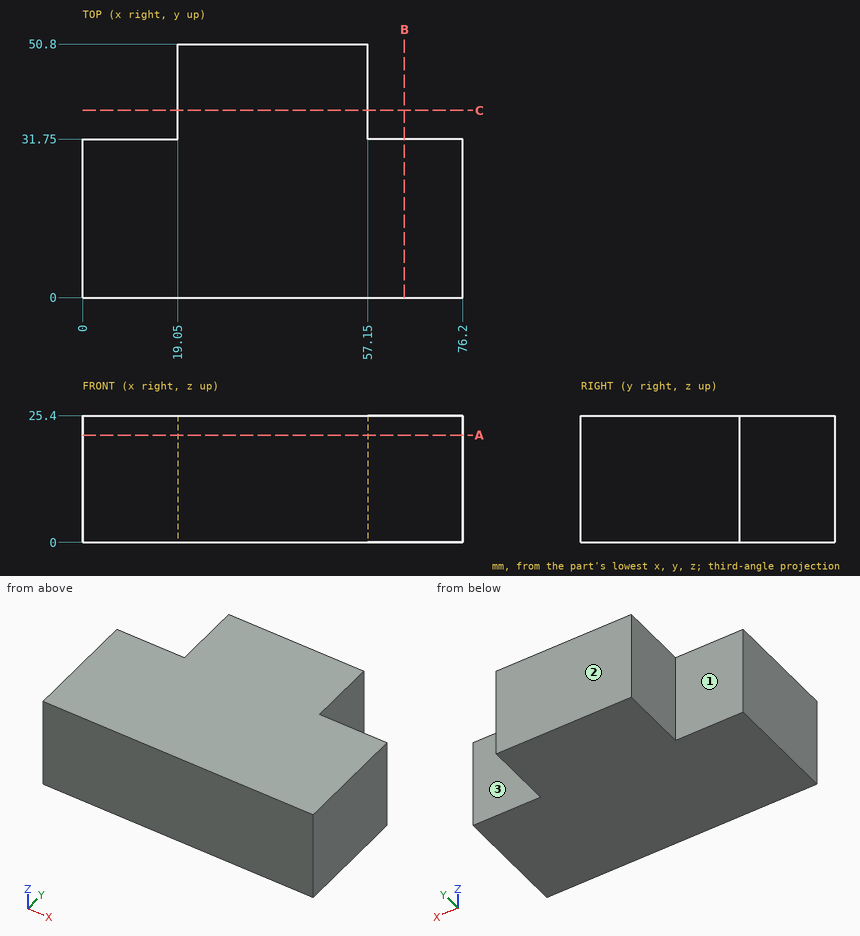
Here's the drawing with two shaded views (mm, measured from the low corner). I have some questions. A direction names the side the tool comes from. Coordinates: 2 decimals unless noted, no trailing zeros. Loops run counter-clockwise (first coordinate to the right, second up) from the corner with the lowest first, then second, coordinate; pieces in that order, holes last. Notation, with made-up numbers: (73.5, -35) -> (101.5, -35) arc R14 cw to (101.5, -18) -> close; hole circle Ø10 at (42, 30.25). An arc over 180 degrees is marked (long way). Answer in a Markdown table with one row per item.
(1) Imagine slicing it at A-A (z = 21.5). List the corners of the cut face in (x, y) for me, plus the area to 3 significant figures.
Results found:
| item | result |
|---|---|
| outline | (0, 0) -> (76.2, 0) -> (76.2, 31.75) -> (57.15, 31.75) -> (57.15, 50.8) -> (19.05, 50.8) -> (19.05, 31.75) -> (0, 31.75) -> close |
| area | 3,150 mm^2 |
(2) For the marked faces 1, 2 and 3, which set-ups out of +Z, -Z, +X, -X, +Y, -Y let a thin tool reach every point of the face, with its end or its side?
Results found:
| item | result |
|---|---|
| face 1 | +Z, -Z, -X, +Y |
| face 2 | +Z, -Z, +X, -X, +Y |
| face 3 | +Z, -Z, +X, +Y |
(3) Imagine slicing it at C-C (y = 37.5). List the corners of the cut face in (x, z) for me, plus the area to 3 significant figures.
Results found:
| item | result |
|---|---|
| outline | (19.05, 0) -> (57.15, 0) -> (57.15, 25.4) -> (19.05, 25.4) -> close |
| area | 968 mm^2 |
(4) If I drill on probe 1 along Y at (x, z) = (68, 3.75); probe 2 along X at (y, z) = (47.5, 9.25), over which ranges is the centre line in solid material (lowest first)?
Results found:
| item | result |
|---|---|
| probe 1 | y = 0 to 31.75 |
| probe 2 | x = 19.05 to 57.15 |
(5) Will these pins go through, and if not, where does the flat tip stop? pin 1 Ø9.5 at (y, z) = (38.5, 12) entering from -X; pin 2 Ø5.5 at (y, z) = (37.5, 6.5) entering from +X; pin 3 Ø9.5 at (x, z) = (8, 6.5) entering from +Y.
Results found:
| item | result |
|---|---|
| pin 1 | stops at x = 19.05 |
| pin 2 | stops at x = 57.15 |
| pin 3 | stops at y = 31.75 |
(6) Imagine slicing it at B-B (x = 64.5). List the corners of the cut face in (y, z) for me, plus the area to 3 significant figures.
Results found:
| item | result |
|---|---|
| outline | (0, 0) -> (31.75, 0) -> (31.75, 25.4) -> (0, 25.4) -> close |
| area | 806 mm^2 |
